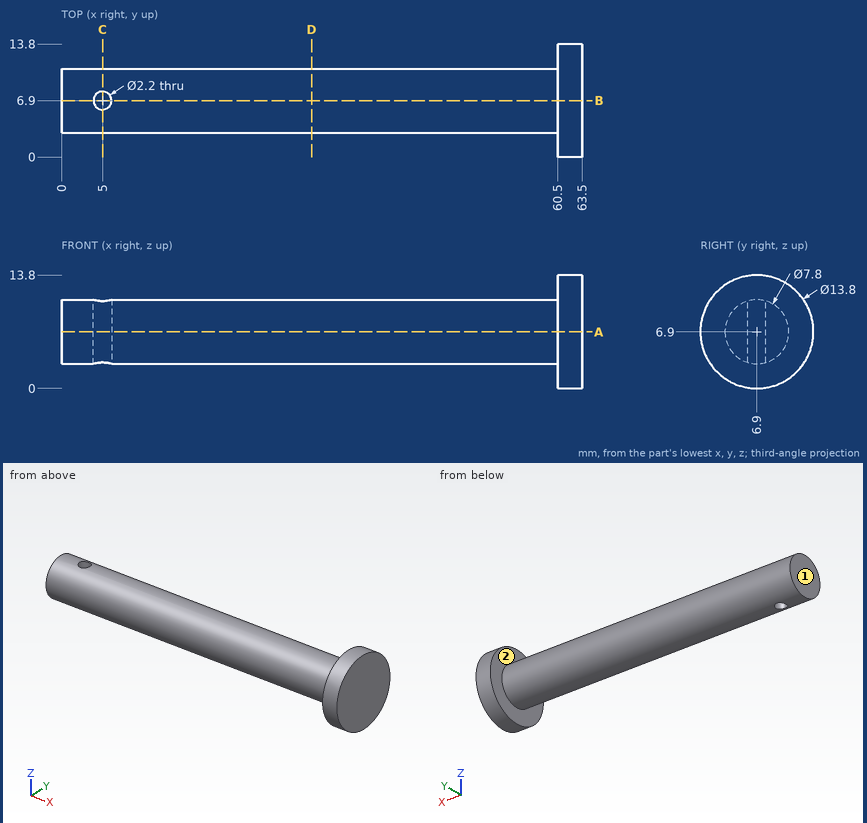
Can you work these out from the drawing? Everything is in mm from the part's minimum corner. A direction names the side the tool comes from. Coordinates: 2 decimals unless noted, no trailing zeros. Loops run counter-clockwise (first coordinate to the right, second up) from the corner with the lowest first, then second, coordinate; pieces in that order, holes last.
1) Imagine slicing it at B-B (y = 6.9). List the corners of the cut face in (x, z) for me.
Reported:
outline: (0, 3) - (3.9, 3) - (3.9, 10.8) - (0, 10.8) - close; (6.1, 3) - (60.5, 3) - (60.5, 0) - (63.5, 0) - (63.5, 13.8) - (60.5, 13.8) - (60.5, 10.8) - (6.1, 10.8) - close
2) Please list where these lines run through material, in increasing order: line 1 along X through (y, z) = (6.9, 9); line 2 along Y through (x, z) = (5, 7); line 3 along X through (y, z) = (11.5, 2).
Reported:
line 1: x = 0 to 3.9, 6.1 to 63.5
line 2: y = 3 to 5.8, 8 to 10.8
line 3: x = 60.5 to 63.5
3) Which directions (+Z, -Z, +X, -X, +Y, -Y) give clear straight access to the entire face, cutting with the end or side of a thin tool? Please do the marked faces 1 and 2.
Reported:
face 1: +Z, -Z, -X, +Y, -Y
face 2: -X
4) Imagine slicing it at D-D (x = 30.5). List the corners of the cut face in (y, z) for me.
Reported:
outline: circle Ø7.8 at (6.9, 6.9)
5) Imagine slicing it at C-C (x = 5). List the corners of the cut face in (y, z) for me, and give its area (3 significant figures).
Reported:
outline: (5.8, 3.16) - (5.8, 10.64) arc R3.9 ccw to start; (8, 3.16) arc R3.9 ccw to (8, 10.64) - close
area: 30.9 mm2
6) Will these pins go through, and if not, where does the flat tip stop? pin 1 Ø3 at (x, y) = (5, 6.9) entering from -Z; pin 2 Ø8 at (x, z) = (29.5, 8) entering from +Y; pin 3 Ø8 at (x, z) = (9.5, 7.5) entering from -Y; pin 4 Ø8 at (y, z) = (6.5, 12) entering from -X.
Reported:
pin 1: stops at z = 3
pin 2: stops at y = 10.8
pin 3: stops at y = 3
pin 4: stops at x = 0
7) Imagine slicing it at A-A (z = 6.9). List the corners of the cut face in (x, y) for me.
Reported:
outline: (0, 3) - (60.5, 3) - (60.5, 0) - (63.5, 0) - (63.5, 13.8) - (60.5, 13.8) - (60.5, 10.8) - (0, 10.8) - close; hole circle Ø2.2 at (5, 6.9)
